Design review of the part built by this model. Coordinates are the model's own, in mm. Coordinates: 2 decimals unless noted, no trailing zeros. Order: outer loops, then holes, each group sorted by start corner. A loop starts at its lowest first (then second) coordinate and runs counter-clockwise, first axis right, second up. Notation, with made-up numbers: (2.25, 21) -> (25.25, 21) arc R25 cw to (25.25, 39) -> close; hole circle Ø2 at (-3.5, 74). An arc over 180 degrees is marked (long way). Use a Markdown table: item, result. Add a question column.
Q1. Add section A-A (x = 3). State the section outline as (y, z) points (3 decimals), then the cut area to 3 significant figures.
Q2. Wall thickness on probe 1 along Y at (x, z) = (326.5, 64); probe 2 along Z at (x, y) = (-40.5, -9.25); probe 3 along Z at (x, y) = (138.5, -17.5): over which ranges is each line inside the solid? List them lowest first.
Q3. Insertion check: pin 1 (8 mm diameter, centred on x = 258.5, y = -11.5, fed in from +Z); pin 2 (3 mm diameter, centred on x = 176.5, y = -2.5, fed in from +Z). Each pin has a flat end and moves straight along its axis. Give the tip position at first contact, or say it passes through.
Q4. Add section B-B (y = -15). State the section outline as (x, z) points, then the cut area to 3 significant figures.
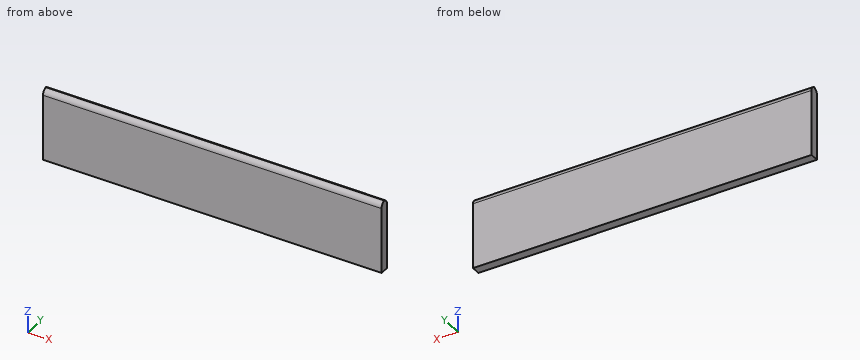
from build123d import *

# Parameters (mm, degrees)
F0_W        = 723.9
F0_H        = 152.4
F1_DEPTH    = 19.05
F2_T1_DEPTH = 787.4


# Not quite as in the source:
# - a fillet or chamfer that OpenCascade refuses, or shapes differently, is made with other operations: its cross-section is extruded or revolved along the edge and cut away or added


with BuildPart() as f1:
    # F0 (on Front) → F1 (new body)
    with BuildSketch(Plane.XZ):
        Rectangle(F0_W, F0_H)
    extrude(amount=F1_DEPTH)

    # F2: fillet of radius 12.7 on 2 edges, made by hand

    # F2_s2 → F2_t1 (cut)
    with BuildSketch(Plane.YZ.offset(-393.7)):
        with BuildLine():
            ThreePointArc((-12.7, 76.2), (-3.7197438789, 72.4802561211), (0, 63.5))
            Line((0, 63.5), (0, 76.2))
            Line((0, 76.2), (-12.7, 76.2))
        make_face()
        with BuildLine():
            ThreePointArc((-6.35, 76.2), (-15.3302561211, 72.4802561211), (-19.05, 63.5))
            Line((-19.05, 63.5), (-19.05, 76.2))
            Line((-19.05, 76.2), (-6.35, 76.2))
        make_face()
    extrude(amount=F2_T1_DEPTH, mode=Mode.SUBTRACT)


solid = f1.part
Established:
| question | item | result |
|---|---|---|
| 1 | outline | (-19.05, -76.2) -> (0, -76.2) -> (0, 63.5) arc R12.7 ccw to (-9.525, 75.797) arc R12.7 ccw to (-19.05, 63.5) -> close |
| 1 | area | 2,830 mm^2 |
| 2 | probe 1 | -19.04 to -0.01 |
| 2 | probe 2 | -76.2 to 75.72 |
| 2 | probe 3 | -76.2 to 69.58 |
| 3 | pin 1 | z = 75.8 |
| 3 | pin 2 | z = 72.75 |
| 4 | outline | (-361.95, -76.2) -> (361.95, -76.2) -> (361.95, 72.8) -> (-361.95, 72.8) -> close |
| 4 | area | 108,000 mm^2 |
